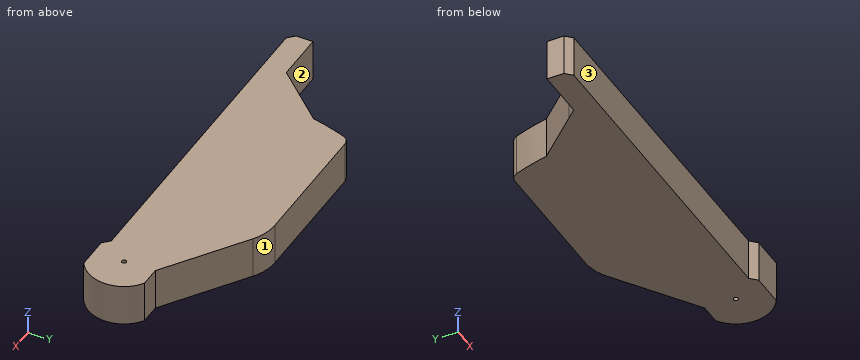
from build123d import *

# Parameters (mm, degrees)
F0_R     = 1.925
F0_W     = 1.25
F0_H     = 2.5
F0_R_2   = 0.5
F1_DEPTH = 9


with BuildPart() as f1:
    # F0 (on Top) → F1 (new body)
    with BuildSketch(Plane.XY):
        Polygon((-35.75, 1.414214), (-34.335786, 0), (-29.522136, 0), (-25.05, 5), (-35.75, 5), align=None)
        with BuildLine():
            Line((-25.05, 5), (-29.522136, 0))
            Line((-29.522136, 0), (-0.75, 0))
            Line((-0.75, 0), (-0.75, 4))
            ThreePointArc((-0.75, 4), (-1.62868, 6.12132), (-3.75, 7))
            Line((-3.75, 7), (-23.261146, 7))
            Line((-23.261146, 7), (-25.05, 5))
        make_face()
        with BuildLine():
            Line((-0.75, 4), (-0.75, 0))
            Line((-0.75, 0), (35.75, 0))
            Line((35.75, 0), (37.164214, -1.414214))
            Line((37.164214, -1.414214), (44.164214, -1.414214))
            ThreePointArc((44.164214, -1.414214), (47.796382, 5.085786), (44.164214, 11.585786))
            Line((44.164214, 11.585786), (39.841021, 11.585786))
            Line((39.841021, 11.585786), (22.611781, 23.275177))
            ThreePointArc((22.611781, 23.275177), (19.934069, 24.559073), (16.997385, 25))
            Line((16.997385, 25), (2.247385, 25))
            Line((2.247385, 25), (2.247385, 22.5))
            Line((2.247385, 22.5), (0.997385, 22.5))
            Line((0.997385, 22.5), (0.997385, 25))
            Line((0.997385, 25), (-11.114516, 25))
            ThreePointArc((-11.114516, 25), (-12.272269, 24.63083), (-13.002615, 23.659607))
            ThreePointArc((-13.002615, 23.659607), (-14.155189, 19.955254), (-15.05, 16.18034))
            Line((-15.05, 16.18034), (-23.261146, 7))
            Line((-23.261146, 7), (-3.75, 7))
            ThreePointArc((-3.75, 7), (-1.62868, 6.12132), (-0.75, 4))
        make_face()
        with Locations((40.164214, 5.085786)):
            Circle(F0_R, mode=Mode.SUBTRACT)
        with Locations((1.622385, 23.75)):
            Rectangle(F0_W, F0_H)
        with Locations((40.164214, 5.085786)):
            Circle(F0_R)
        with Locations((40.164214, 5.085786)):
            Circle(F0_R_2, mode=Mode.SUBTRACT)
    extrude(amount=F1_DEPTH)


solid = f1.part
Geometry check sheet. Reference: the model listing, model coordinates, mm. Face numbers are marked on the shaded views. A direction names the side the tool comes from. Give positions to 0.01 mm unless a question says otherwise; leave off trailing zeros. Loops run counter-clockwise (first coordinate to the right, second up) from the corner with the lowest first, then second, coordinate; pieces in that order, holes last. Notation, with made-up numbers: (-13, -12.75) -> (34, -12.75) arc R31 ccw to (34, 25.25) -> close; hole circle Ø5 at (-35, 33). An arc over 180 degrees is marked (long way). Answer in a Markdown table with one row per item. Add a question column.
1) Material ranges on probe 1 along Y at (x, z) = (5, 1); probe 2 along Y at (x, z) = (43, 5.75); probe 3 along X at (y, z) = (11, 7), recorded low to high. Write a range as from..to.
2) Cross-section at B-B on x = 42.5. Record the boundary of the cut face in (y, z), and give its area (3 significant figures).
3) Cross-section at C-C on y = 7.75. Record the boundary of the cut face in (x, z).
4) Cross-section at A-A on z = 5.25. Record the boundary of the cut face in (x, y).
5) Gauge pin test, flat ends, axial feed: P1, Ø3.5, axis at x = 42.5, z = 3.5, coming from the +Y side; P2, Ø5, axis at y = 2, z = 7.5, coming from the +X side; P3, Ø2.5, axis at x = -11, z = 3, coming from the -Y side. Record the tip position at first contact, or that the pin passes through.
6) Set-up check for the marked faces 1, 2 and 3: record each of +Z, -Z, +X, -X, +Y, -Y from which the full face is reachable in a straight line by a thin tool's end or side.
Outcome:
| question | item | result |
|---|---|---|
| 1 | probe 1 | y = 0..25 |
| 1 | probe 2 | y = -1.41..11.59 |
| 1 | probe 3 | x = -19.68..44.99 |
| 2 | outline | (-1.41, 0) -> (11.59, 0) -> (11.59, 9) -> (-1.41, 9) -> close |
| 2 | area | 117 mm^2 |
| 3 | outline | (-22.59, 0) -> (47.32, 0) -> (47.32, 9) -> (-22.59, 9) -> close |
| 4 | outline | (-35.75, 1.41) -> (-34.34, 0) -> (35.75, 0) -> (37.16, -1.41) -> (44.16, -1.41) arc R7.63 ccw to (44.16, 11.59) -> (39.84, 11.59) -> (22.61, 23.28) arc R10 ccw to (17, 25) -> (-11.11, 25) arc R2 ccw to (-13, 23.66) arc R56.32 ccw to (-15.05, 16.18) -> (-23.26, 7) -> (-25.05, 5) -> (-35.75, 5) -> close; hole circle Ø1 at (40.16, 5.09) |
| 5 | P1 | stops at y = 11.59 |
| 5 | P2 | stops at x = 47.77 |
| 5 | P3 | stops at y = 0 |
| 6 | face 1 | +Z, -Z, +X, +Y |
| 6 | face 2 | +Z, -Z, -X, +Y |
| 6 | face 3 | +Z, -Z, -X, -Y |
